For this review, use the dimensioned drawing (mm, ordinates from the lowest corner) and the shaded views. A direction names the side the tool comes from. Round coordinates to 2 decimals unless told otherwise and drop trailing zeros. Write each loop counter-clockwise with the first axis right and the second up, starting at its lowest first coordinate (ties: lowest second). Pieces come first, ordered by that corner, then holes. Notation, with made-up numbers: M 35.25,-9 L 53.25,-9 A26 ccw 53.25,5 Z; hole C -10.75,24 d11. An arc over 180 degrees is marked long. Use one line per item in the form item = value. Start each with the question number.
Item 1: For line 1 (X direction, y = 1.55, z = 52.5); line 2 (Z direction, x = 47, y = 1.25); line 3 (X direction, y = 0.55, z = 34), list the stretches that pass through material, from the lowest coordinate up. Write a range as [from, to].
Item 2: For P1, Ø0.5, axis at y = 1.5, z = 20, coming from the +X side; P2, Ø1.1, axis at y = 1.5, z = 87.5, coming from the -X side; P3, Ø3, axis at x = 50, z = 87.5, coming from the +Y side, all flat-tipped, find the tip position at first contact; note any pin that passes through.
Item 3: Draft analysis for pull direction Z (two halves, no side actions). For the marked faces 3 and 4, state which applies: released by +Z, released by -Z, zero draft, split by the parting line, or undercut.
Item 4: Add section A-A (y = 1.5). State the section outline as (x, z) points, and give its area (3 significant figures).
Item 5: For the marked faces 1 and 2, list the 3-axis set-ups (+Z, -Z, +X, -X, +Y, -Y) from which the entire face can be reached by the end or side of a thin tool; tool diameter is ignored.
Item 6: Add section D-D (z = 87.5). State the section outline as (x, y) points, and give its area (3 significant figures).
Item 7: Add section B-B (z = 54). State the section outline as (x, y) points, and give its area (3 significant figures).
Item 8: Add section C-C (x = 54). State the section outline as (y, z) points, and give its area (3 significant figures).
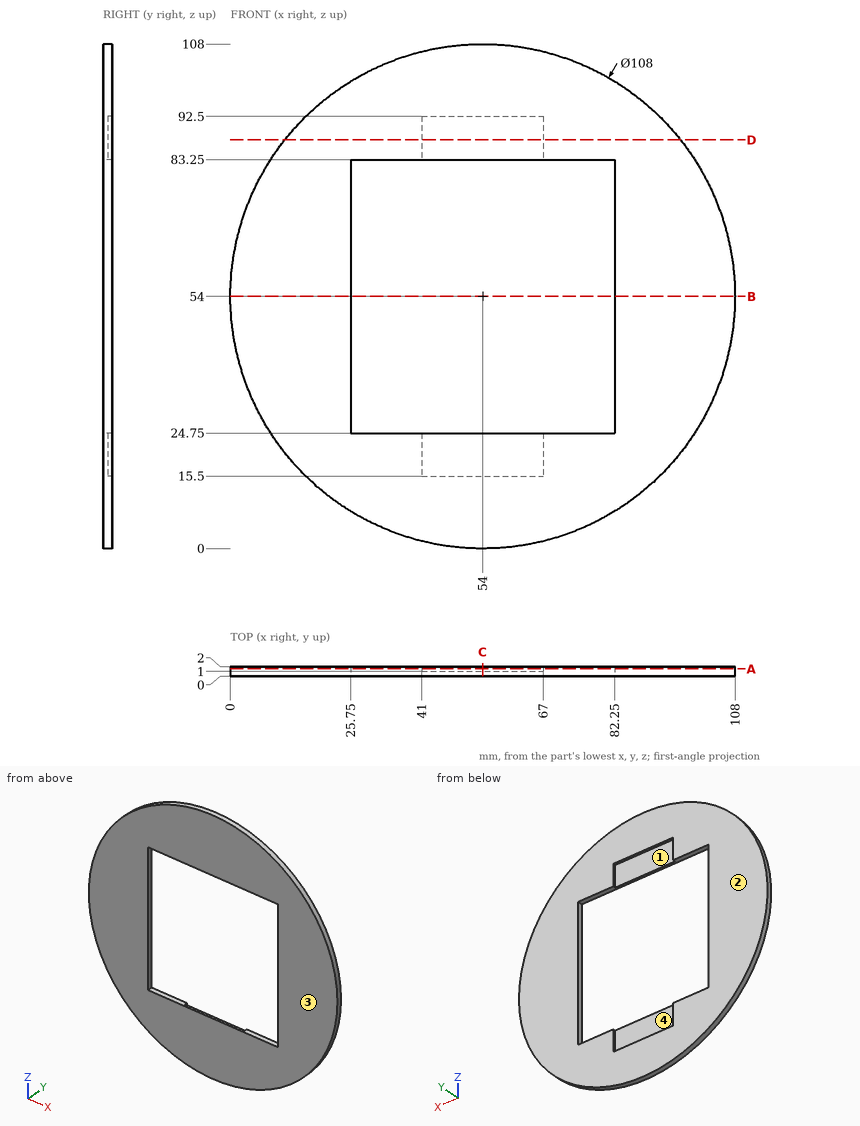
Calculated:
q1.line_1 = [0.02, 25.75], [82.25, 107.98]
q1.line_2 = [0.46, 15.5], [92.5, 107.54]
q1.line_3 = [3.84, 25.75], [82.25, 104.16]
q2.P1 = 96.15
q2.P2 = 11.22
q2.P3 = 1
q3.face_3 = zero draft
q3.face_4 = undercut
q4.outline = C 54,54 d108; hole M 25.75,24.75 L 41,24.75 L 41,15.5 L 67,15.5 L 67,24.75 L 82.25,24.75 L 82.25,83.25 L 67,83.25 L 67,92.5 L 41,92.5 L 41,83.25 L 25.75,83.25 Z
q4.area = 5,370 mm^2
q5.face_1 = +Y
q5.face_2 = +Z, -Z, +X, -X, +Y
q6.outline = M 11.65,0 L 96.35,0 L 96.35,2 L 67,2 L 67,1 L 41,1 L 41,2 L 11.65,2 Z
q6.area = 143 mm^2
q7.outline = M 0,0 L 25.75,0 L 25.75,2 L 0,2 Z; M 82.25,0 L 108,0 L 108,2 L 82.25,2 Z
q7.area = 103 mm^2
q8.outline = M 0,0 L 2,0 L 2,15.5 L 1,15.5 L 1,24.75 L 0,24.75 Z; M 0,83.25 L 1,83.25 L 1,92.5 L 2,92.5 L 2,108 L 0,108 Z
q8.area = 80.5 mm^2
